from build123d import *

# Parameters (mm, degrees)
SKETCH1_W           = 21.59
SKETCH1_H           = 81.67214734
BOSS_EXTRUDE1_DEPTH = 6.35
SKETCH2_W           = 21.59
SKETCH2_H           = 15.68610503
CUT_EXTRUDE1_DEPTH  = 6.35
SKETCH3_R           = 1.524
CUT_EXTRUDE2_DEPTH  = 6.35


with BuildPart() as part:
    # Sketch1 → Boss-Extrude1 (new body)
    with BuildSketch(Plane(origin=(0, 0, 0), x_dir=(1, 0, 0), z_dir=(0, 1, 0))):
        Rectangle(SKETCH1_W, SKETCH1_H)
    extrude(amount=BOSS_EXTRUDE1_DEPTH)

    # Sketch2 → Cut-Extrude1 (cut)
    with BuildSketch(Plane(origin=(0, 6.35, 0), x_dir=(1, 0, 0), z_dir=(0, 1, 0))):
        with Locations((0, -32.993021155)):
            Rectangle(SKETCH2_W, SKETCH2_H)
    extrude(amount=-CUT_EXTRUDE1_DEPTH, mode=Mode.SUBTRACT)

    # Sketch3 → Cut-Extrude2 (cut)
    with BuildSketch(Plane(origin=(0, 6.35, 0), x_dir=(1, 0, 0), z_dir=(0, 1, 0))):
        with Locations(Location((0, 28.13607367, 0), (0, 0, 270))):
            Circle(SKETCH3_R)
    extrude(amount=-CUT_EXTRUDE2_DEPTH, mode=Mode.SUBTRACT)


solid = part.part
Read the model definition and answer for the solid it produces. Units are mm, in the model's axes. Give positions to 0.01 mm unless a question says otherwise; leave off trailing zeros. Write each loop counter-clockwise with the first axis right and the second up, starting at its lowest first coordinate (ties: lowest second). Pieces come first, ordered by that corner, then holes. Notation, with made-up numbers: M -9,54.25 L 35,54.25 A27 cw 35,72.25 Z; hole C -19.5,0 d4. An arc over 180 degrees is marked long. One line per item, written item: value. Start each with the question number.
(1) A flat-ended cylindrical pin translates along its axis: pin 1 Ø2.5 at (x, z) = (0, -28.14) entering from -Y. Find the tip coordinate at first contact, or state that the pin passes through.
(2) Find the intervals of material crossed by line 1 (Z direction, x = -0.5, y = 3.5); line 2 (Z direction, x = -1, y = 1.5), in increasing order.
(3) Determine the mould class of faces 1 (the flat face through (0, 3, 25.15)), 2 (the flat face through (-10.795, 3, -7)), 3 (the cylindrical face through (0.458, 3.219, -26.682)), 4 (the flat face through (10.795, 3, -7)) for opening direction X: pulls with the +X half, pulls with the -X half, needs draft (parallel to the pull), parting line crosses it, or undercut.
(4) Find section B-B (z = -28). Determine the outline of the cut face in (x, y) (3 decimals).
(5) Find section A-A (x = 0). Determine the outline of the cut face in (y, z), plus the area to 3 significant figures.
Results below:
1. pin 1: passes through
2. line 1: z = -40.84 to -29.58, -26.7 to 25.15
2. line 2: z = -40.84 to -29.29, -26.99 to 25.15
3. face 1: needs draft
3. face 2: pulls with the -X half
3. face 3: undercut
3. face 4: pulls with the +X half
4. outline: M -10.795,0 L -1.518,0 L -1.518,6.35 L -10.795,6.35 Z; M 1.518,0 L 10.795,0 L 10.795,6.35 L 1.518,6.35 Z
5. outline: M 0,-40.84 L 6.35,-40.84 L 6.35,-29.66 L 0,-29.66 Z; M 0,-26.61 L 6.35,-26.61 L 6.35,25.15 L 0,25.15 Z
5. area: 400 mm^2
